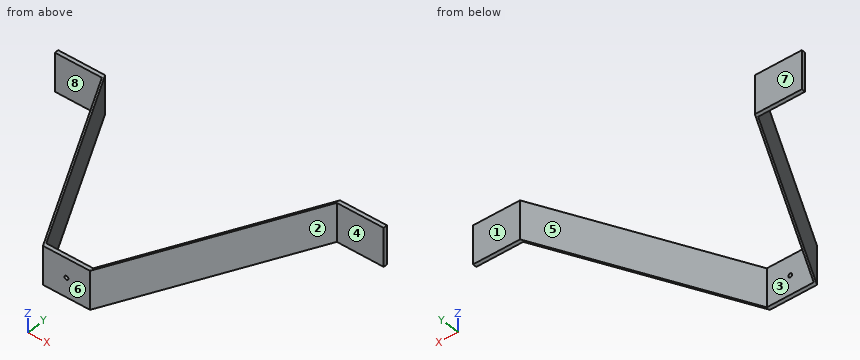
from build123d import *

# Parameters (mm, degrees)
SKETCH1_W           = 76.2
SKETCH1_H           = 63.5
BOSS_EXTRUDE1_DEPTH = 6.35
SKETCH2_R           = 3.175
CUT_EXTRUDE1_DEPTH  = 50.99995
BOSS_EXTRUDE2_DEPTH = 63.5
SKETCH4_W           = 63.5
SKETCH4_H           = 6.35
BOSS_EXTRUDE3_DEPTH = 76.2


with BuildPart() as part:
    # Sketch1 → Boss-Extrude1 (new body)
    with BuildSketch(Plane(origin=(0, 0, 0), x_dir=(1, 0, 0), z_dir=(0, 1, 0))):
        Rectangle(SKETCH1_W, SKETCH1_H)
    extrude(amount=BOSS_EXTRUDE1_DEPTH)

    # Sketch2 → Cut-Extrude1 (cut, through all)
    with BuildSketch(Plane(origin=(0, 6.35, 0), x_dir=(1, 0, 0), z_dir=(0, 1, 0))):
        with Locations(Location((0, 0, 0), (0, 0, 270))):
            Circle(SKETCH2_R)
    extrude(amount=-CUT_EXTRUDE1_DEPTH, mode=Mode.SUBTRACT)

    # Sketch3 → Boss-Extrude2 (add)
    with BuildSketch(Plane.XY.offset(31.75)):
        Polygon((38.1, 6.35), (190.5, 304.8), (190.5, 298.45), (38.1, 0), align=None)
    boss_extrude2 = extrude(amount=-BOSS_EXTRUDE2_DEPTH)

    # Sketch4 → Boss-Extrude3 (add)
    with BuildSketch(Plane(origin=(190.5, 0, 0), x_dir=(0, 0, -1), z_dir=(1, 0, 0))):
        with Locations((0, 301.625)):
            Rectangle(SKETCH4_W, SKETCH4_H)
    boss_extrude3 = extrude(amount=BOSS_EXTRUDE3_DEPTH)

    # Mirror1: Boss-Extrude2, Boss-Extrude3 across plane
    add(boss_extrude2.mirror(Plane(origin=(0, 0, 0), x_dir=(0, 0, 1), z_dir=(1, 0, 0))))
    add(boss_extrude3.mirror(Plane(origin=(0, 0, 0), x_dir=(0, 0, 1), z_dir=(1, 0, 0))))


solid = part.part
Design review of the part built by this model. Coordinates are the model's own, in mm. Face numbers are marked on the shaded views. A direction names the side the tool comes from. Coordinates: 2 decimals unless noted, no trailing zeros. Order: outer loops, then holes, each group sorted by start corner. A loop starts at its lowest first (then second) coordinate and runs counter-clockwise, first axis right, second up. Notation, with made-up numbers: M -7,88.25 L -3,88.25 A4 cw -3,95.25 Z; hole C 62.5,-15.5 d4. An arc over 180 degrees is marked long. Use a Markdown table: item, result.
(1) Wall thickness on probe 1 along X at (y, z) = (174.5, -15); probe 2 along X at (y, z) = (208.5, -9); probe 3 along Y at (x, z) = (234, -18): over which ranges is each line inside the solid? List them lowest first.
Worked answers:
| item | result |
|---|---|
| probe 1 | x = -127.21 to -123.96, 123.96 to 127.21 |
| probe 2 | x = -144.57 to -141.33, 141.33 to 144.57 |
| probe 3 | y = 298.45 to 304.8 |
(2) For the marked faces 4, 5, 6, 7 and 8, list the 3-axis set-ups (+Z, -Z, +X, -X, +Y, -Y) from which the entire face can be reached by the end or side of a thin tool; tool diameter is ignored.
Worked answers:
| item | result |
|---|---|
| face 4 | +Z, -Z, +X, -Y |
| face 5 | +Z, -Z, +Y |
| face 6 | +Z, -Z, +X, -X, -Y |
| face 7 | +Z, -Z, +X, -X, +Y |
| face 8 | +Z, -Z, -X, -Y |
(3) Add section C-C (x = 54). Give the boundary of the cut face in (y, z), then the cut area to 3 significant figures.
Worked answers:
| item | result |
|---|---|
| outline | M 31.14,-31.75 L 37.49,-31.75 L 37.49,31.75 L 31.14,31.75 Z |
| area | 403 mm2 |
(4) Add section A-A (y = 102). Give the boundary of the cut face in (x, z), then the cut area to 3 significant figures.
Worked answers:
| item | result |
|---|---|
| outline | M -90.19,-31.75 L -86.94,-31.75 L -86.94,31.75 L -90.19,31.75 Z; M 86.94,-31.75 L 90.19,-31.75 L 90.19,31.75 L 86.94,31.75 Z |
| area | 412 mm2 |
(5) For P1, Ø19, axis at x = 210.5, z = -15.5, coming from the -Y side; P2, Ø4, axis at x = 118, z = -17, coming from the -Y side; P3, Ø1, axis at y = 145, z = 6.5, coming from the -X side, all flat-tipped, find the tip position at first contact; note any pin that passes through.
Worked answers:
| item | result |
|---|---|
| P1 | stops at y = 298.45 |
| P2 | stops at y = 152.55 |
| P3 | stops at x = -112.4 |
(6) Draft analysis for pull direction X (two halves, no side actions). For the marked faces 1, 2 and 3, state which applies: released by +X, released by -X, zero draft, split by the parting line, or undercut.
Worked answers:
| item | result |
|---|---|
| face 1 | zero draft |
| face 2 | released by +X |
| face 3 | undercut |
(7) Add section B-B (z = -9). Give the boundary of the cut face in (x, y).
Worked answers:
| item | result |
|---|---|
| outline | M -266.7,298.45 L -190.5,298.45 L -38.1,0 L 38.1,0 L 190.5,298.45 L 266.7,298.45 L 266.7,304.8 L 190.5,304.8 L 38.1,6.35 L -38.1,6.35 L -190.5,304.8 L -266.7,304.8 Z |
